Model file for the job. Use its own axes, mm. Round coordinates to 2 decimals unless told otherwise and drop trailing zeros. Loops run counter-clockwise (first coordinate to the right, second up) from the corner with the lowest first, then second, coordinate; pieces in that order, holes last. Notation, with made-up numbers: (47, 8.5) - (69, 8.5) arc R30 ccw to (69, 36.5) - close; hole circle Ø1 at (-30, -12.75). An arc over 180 degrees is marked (long way). Answer as a JSON object with one key per item and string values.
from build123d import *

# Parameters (mm, degrees)
BOSS_EXTRUDE1_DEPTH = 3
SKETCH2_R           = 10
SKETCH2_W           = 3
SKETCH2_H           = 56
SKETCH2_W_2         = 40
SKETCH2_H_2         = 3
CUT_EXTRUDE1_DEPTH  = 166.830173222


with BuildPart() as part:
    # Sketch1 → Boss-Extrude1 (new body)
    with BuildSketch(Plane(origin=(0, 0, 0), x_dir=(1, 0, 0), z_dir=(0, 1, 0))):
        Polygon((15.838364304, 121), (55.838364304, 121), (55.838364304, 118), (92.838364304, 118), (92.838364304, 73), (95.838364304, 73), (95.838364304, 23), (92.838364304, 23), (92.838364304, -31), (95.838364304, -31), (95.838364304, -81), (92.838364304, -81), (92.838364304, -126), (55.838364304, -126), (55.838364304, -129), (15.838364304, -129), (15.838364304, -126), (-24.161635696, -126), (-24.161635696, -129), (-64.161635696, -129), (-64.161635696, -126), (-101.161635696, -126), (-101.161635696, -81), (-104.161635696, -81), (-104.161635696, -31), (-101.161635696, -31), (-101.161635696, 23), (-104.161635696, 23), (-104.161635696, 73), (-101.161635696, 73), (-101.161635696, 118), (-64.161635696, 118), (-64.161635696, 121), (-24.161635696, 121), (-24.161635696, 118), (15.838364304, 118), align=None)
    extrude(amount=BOSS_EXTRUDE1_DEPTH)

    # Sketch2 → Cut-Extrude1 (cut, through all)
    with BuildSketch(Plane(origin=(0, 3, 0), x_dir=(1, 0, 0), z_dir=(0, 1, 0))):
        with Locations(Location((-4.300530568, 0, 0), (0, 0, 270))):
            Circle(SKETCH2_R)
        with Locations(Location((35.699469432, 0, 0), (0, 0, 270))):
            Circle(SKETCH2_R)
        with Locations(Location((75.699469432, 0, 0), (0, 0, 270))):
            Circle(SKETCH2_R)
        with Locations(Location((-44.300530568, 0, 0), (0, 0, 270))):
            Circle(SKETCH2_R)
        with Locations(Location((-84.300530568, 0, 0), (0, 0, 270))):
            Circle(SKETCH2_R)
        with Locations(Location((-84.300530568, 50, 0), (0, 0, 270))):
            Circle(SKETCH2_R)
        with Locations(Location((-44.300530568, 50, 0), (0, 0, 270))):
            Circle(SKETCH2_R)
        with Locations(Location((-4.300530568, 50, 0), (0, 0, 270))):
            Circle(SKETCH2_R)
        with Locations(Location((35.699469432, 50, 0), (0, 0, 270))):
            Circle(SKETCH2_R)
        with Locations(Location((75.699469432, 50, 0), (0, 0, 270))):
            Circle(SKETCH2_R)
        with Locations(Location((-84.300530568, 100, 0), (0, 0, 270))):
            Circle(SKETCH2_R)
        with Locations(Location((-44.300530568, 100, 0), (0, 0, 270))):
            Circle(SKETCH2_R)
        with Locations(Location((-4.300530568, 100, 0), (0, 0, 270))):
            Circle(SKETCH2_R)
        with Locations(Location((35.699469432, 100, 0), (0, 0, 270))):
            Circle(SKETCH2_R)
        with Locations(Location((75.699469432, 100, 0), (0, 0, 270))):
            Circle(SKETCH2_R)
        with Locations(Location((-84.300530568, -50, 0), (0, 0, 270))):
            Circle(SKETCH2_R)
        with Locations(Location((-44.300530568, -50, 0), (0, 0, 270))):
            Circle(SKETCH2_R)
        with Locations(Location((-4.300530568, -50, 0), (0, 0, 270))):
            Circle(SKETCH2_R)
        with Locations(Location((35.699469432, -50, 0), (0, 0, 270))):
            Circle(SKETCH2_R)
        with Locations(Location((75.699469432, -50, 0), (0, 0, 270))):
            Circle(SKETCH2_R)
        with Locations(Location((-84.300530568, -100, 0), (0, 0, 270))):
            Circle(SKETCH2_R)
        with Locations(Location((-44.300530568, -100, 0), (0, 0, 270))):
            Circle(SKETCH2_R)
        with Locations(Location((-4.300530568, -100, 0), (0, 0, 270))):
            Circle(SKETCH2_R)
        with Locations(Location((35.699469432, -100, 0), (0, 0, 270))):
            Circle(SKETCH2_R)
        with Locations(Location((75.699469432, -100, 0), (0, 0, 270))):
            Circle(SKETCH2_R)
        with Locations((-64.161635696, -53)):
            Rectangle(SKETCH2_W, SKETCH2_H)
        Polygon((-65.661635696, 25), (-65.661635696, 81), (-62.661635696, 81), (-62.661635696, 25), (-64.161635696, 25), align=None)
        Polygon((54.338364304, 81), (57.338364304, 81), (57.338364304, 25), (55.838364304, 25), (54.338364304, 25), align=None)
        with Locations((55.838364304, -53)):
            Rectangle(SKETCH2_W, SKETCH2_H)
        with Locations((-4.161635696, 79.5)):
            Rectangle(SKETCH2_W_2, SKETCH2_H_2)
        with Locations((-4.161635696, -79.5)):
            Rectangle(SKETCH2_W_2, SKETCH2_H_2)
    extrude(amount=-CUT_EXTRUDE1_DEPTH, mode=Mode.SUBTRACT)


solid = part.part
1) Two-plate mould, pull along X, no slides. Class faces 1 (the cylindrical face through (-94.063, 1.521, -2.168)), 2 (the flat face through (19, 3, 2)), 3 (the cylindrical face through (-3.86, 1.52, 40.01)): pulls with the +X half, pulls with the -X half, needs draft (parallel to the pull), parting line crosses it, or undercut.
Values follow:
{"face 1": "undercut", "face 2": "needs draft", "face 3": "undercut"}
2) Slice it at A-A on z = -50. Count the separate pieces of the cut face and the enclosed holes in it, then the cut area to 3 significant figures.
Values follow:
{"separate pieces": "8", "enclosed holes": "0", "area": "282 mm²"}
3) Probe probe 1 along X at (y, z) = (0.65, 34); probe 2 along Z at (x, y) = (-64, 1.1); probe 3 along Z at (x, y) = (-19, 0.7). List the from-to ranges inside material, lowest first.
Values follow:
{"probe 1": "-104.16 to -65.66, -62.66 to 54.34, 57.34 to 95.84", "probe 2": "-121 to -81, -25 to 25, 81 to 129", "probe 3": "-118 to -81, -78 to 78, 81 to 126"}
4) Drop flat-ended pins along their axis: P1, Ø1.5, axis at x = 2.5, y = 2, coming from the +Z side; P2, Ø0.9, axis at x = -103, y = 1, coming from the -Z side; P3, Ø0.9, axis at x = -80, y = 1.5, coming from the -Z side; P4, Ø16, axis at x = -84.3, z = 50, coming from the -Y side. Give the stop position or say it passes through.
Values follow:
{"P1": "z = 126", "P2": "z = -73", "P3": "z = -118", "P4": "through"}
5) Slice it at B-B on z = 0. List the corners of the cut face in (x, y).
Values follow:
{"outline": "(-101.16, 0) - (-94.3, 0) - (-94.3, 3) - (-101.16, 3) - close; (-74.3, 0) - (-54.3, 0) - (-54.3, 3) - (-74.3, 3) - close; (-34.3, 0) - (-14.3, 0) - (-14.3, 3) - (-34.3, 3) - close; (5.7, 0) - (25.7, 0) - (25.7, 3) - (5.7, 3) - close; (45.7, 0) - (65.7, 0) - (65.7, 3) - (45.7, 3) - close; (85.7, 0) - (92.84, 0) - (92.84, 3) - (85.7, 3) - close"}
